from build123d import *

# Parameters (mm, degrees)
SKETCH1_W           = 71
SKETCH1_H           = 71
SKETCH1_R           = 1.5
SKETCH1_R_2         = 11
SKETCH1_R_3         = 1.631951877
BOSS_EXTRUDE1_DEPTH = 5
FILLET1_R           = 8


with BuildPart() as part:
    # Sketch1 → Boss-Extrude1 (new body)
    with BuildSketch(Plane(origin=(0, 0, 0), x_dir=(0, 0, -1), z_dir=(1, 0, 0))):
        with Locations((35.5, 35.5)):
            Rectangle(SKETCH1_W, SKETCH1_H)
        with Locations((6, 6)):
            Circle(SKETCH1_R, mode=Mode.SUBTRACT)
        with Locations((6, 65)):
            Circle(SKETCH1_R, mode=Mode.SUBTRACT)
        with Locations((65, 65)):
            Circle(SKETCH1_R, mode=Mode.SUBTRACT)
        with Locations((65, 6)):
            Circle(SKETCH1_R, mode=Mode.SUBTRACT)
        with Locations((35.5, 35.5)):
            Circle(SKETCH1_R_2, mode=Mode.SUBTRACT)
        with Locations((25.5, 45.5)):
            Circle(SKETCH1_R_3, mode=Mode.SUBTRACT)
        with Locations((45.5, 45.5)):
            Circle(SKETCH1_R_3, mode=Mode.SUBTRACT)
        with Locations((25.5, 25.5)):
            Circle(SKETCH1_R_3, mode=Mode.SUBTRACT)
        with Locations((45.5, 25.5)):
            Circle(SKETCH1_R_3, mode=Mode.SUBTRACT)
    extrude(amount=BOSS_EXTRUDE1_DEPTH)

    # Fillet1
    fillet1_edges = [part.edges().sort_by_distance(p)[0] for p in [
        (2.5, 71, 0),
        (2.5, 71, -71),
        (2.5, 0, -71),
        (2.5, 0, 0),
    ]]
    fillet(fillet1_edges, radius=FILLET1_R)


solid = part.part
CAD build for the part. Positions are in the model's coordinates, mm. Round coordinates to 2 decimals unless told otherwise and drop trailing zeros. Loops run counter-clockwise (first coordinate to the right, second up) from the corner with the lowest first, then second, coordinate; pieces in that order, holes last. Notation, with made-up numbers: (18, -22) - (42, -22) arc R25 ccw to (42, 7) - close; hole circle Ø3 at (-25, -16.5). An arc over 180 degrees is marked (long way). Put each result on its own line as item: value.
1. Slice it at C-C on y = 6. List the corners of the cut face in (x, z).
Geometry check:
outline: (0, -70.75) - (5, -70.75) - (5, -66.5) - (0, -66.5) - close; (0, -63.5) - (5, -63.5) - (5, -7.5) - (0, -7.5) - close; (0, -4.5) - (5, -4.5) - (5, -0.25) - (0, -0.25) - close
2. Slice it at A-A on z = -35.5. List the corners of the cut face in (x, y).
Geometry check:
outline: (0, 0) - (5, 0) - (5, 24.5) - (0, 24.5) - close; (0, 46.5) - (5, 46.5) - (5, 71) - (0, 71) - close
3. Two-plate mould, pull along Y, no slides. Class faces 1 (the flat face through (2, 0, -35)), 2 (the flat face through (5, 44, -27)), 3 (the cylindrical face through (2.46, 6.45, -66.43)), 4 (the cylindrical face through (2.5, 5.1, -4.8)): released by +Y, released by -Y, zero draft, split by the parting line, or undercut.
Geometry check:
face 1: released by -Y
face 2: zero draft
face 3: undercut
face 4: undercut
4. Slice it at D-D on y = 41. List the corners of the cut face in (x, z), and give its area (3 significant figures).
Geometry check:
outline: (0, -71) - (5, -71) - (5, -45.03) - (0, -45.03) - close; (0, -25.97) - (5, -25.97) - (5, 0) - (0, 0) - close
area: 260 mm²
5. Wall check: line 1 (Y direction, x = 3.2, z = -44); line 2 (Y direction, x = 1.95, z = -25.5); line 3 (Y direction, x = 2.4, z = -6). Give the ranges that are in metal, low to high.
Geometry check:
line 1: 0 to 24.86, 26.14 to 28.52, 42.48 to 44.86, 46.14 to 71
line 2: 0 to 23.87, 27.13 to 30.92, 40.08 to 43.87, 47.13 to 71
line 3: 0.25 to 4.5, 7.5 to 63.5, 66.5 to 70.75
6. Slice it at B-B on x = 3.65. Give the number of separate pieces and of enclosed holes in the cut face, and give its area (3 significant figures).
Geometry check:
separate pieces: 1
enclosed holes: 9
area: 4,540 mm²
